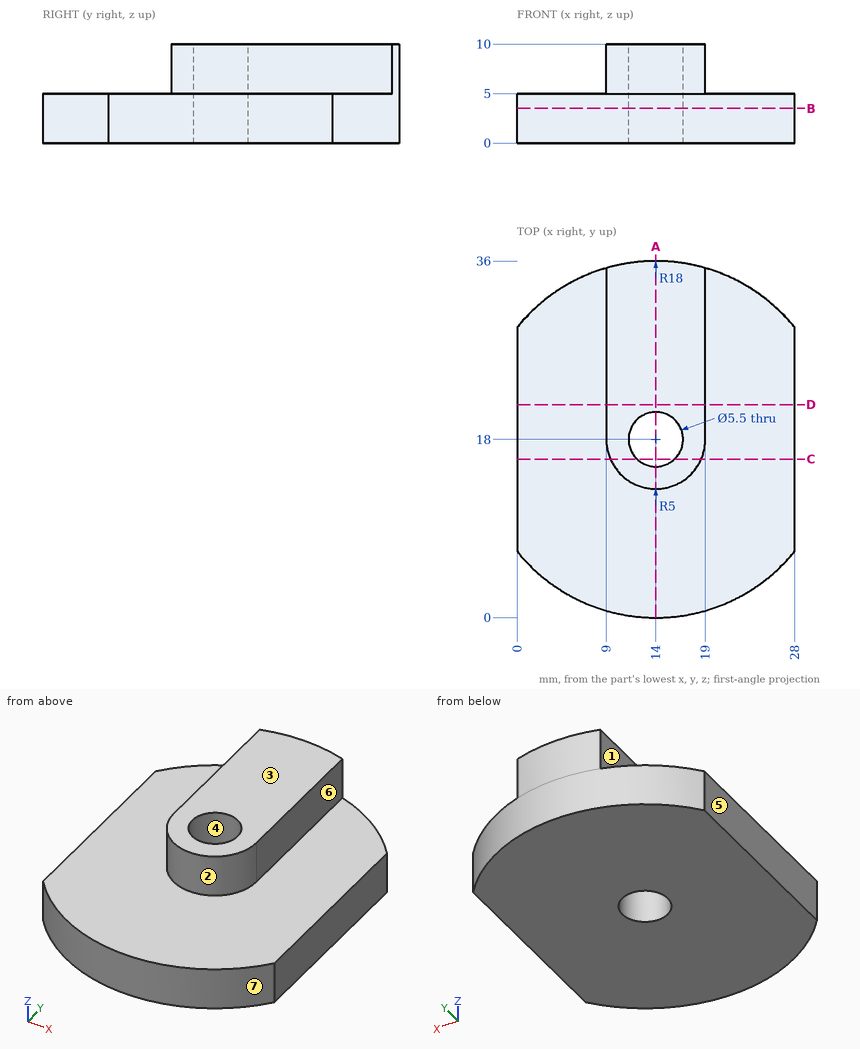
Check sheet for the drawn part. Datum: minimum x, y, z corner. Units: mm. A direction names the side the tool comes from. Round coordinates to 2 decimals unless told otherwise and drop trailing zeros. Order: outer loops, then holes, each group sorted by start corner. A loop starts at its lowest first (then second) coordinate and runs counter-clockwise, first axis right, second up. Notation, with made-up numbers: M 48,46 L 70,46 A14 cw 70,64 Z; hole C -34,23.5 d2. An arc over 180 degrees is marked long. Answer in a Markdown table with one row per item.
(1) Section check D-D on y = 21.5. Record the boundary of the cut face in (x, z), plus the area to 3 significant figures.
Findings:
| item | result |
|---|---|
| outline | M 0,0 L 28,0 L 28,5 L 19,5 L 19,10 L 9,10 L 9,5 L 0,5 Z |
| area | 190 mm^2 |
(2) Material ranges on line 1 along X through (y, z) = (18, 3); line 2 along Y through (x, z) = (14, 2.5); line 3 along Y through (x, z) = (14, 6.25), recorded low to high. Write a range as from..to.
Findings:
| item | result |
|---|---|
| line 1 | x = 0..11.25, 16.75..28 |
| line 2 | y = 0..15.25, 20.75..36 |
| line 3 | y = 13..15.25, 20.75..36 |
(3) Set-up check for the marked faces 1, 2 and 3: record each of +Z, -Z, +X, -X, +Y, -Y from which the full face is reachable in a straight line by a thin tool's end or side.
Findings:
| item | result |
|---|---|
| face 1 | +Z, -X, +Y, -Y |
| face 2 | +Z, -Y |
| face 3 | +Z, +X, -X, +Y, -Y |
(4) Section check C-C on y = 16. Record the boundary of the cut face in (x, z).
Findings:
| item | result |
|---|---|
| outline | M 0,0 L 12.11,0 L 12.11,10 L 9.42,10 L 9.42,5 L 0,5 Z; M 15.89,0 L 28,0 L 28,5 L 18.58,5 L 18.58,10 L 15.89,10 Z |
(5) Section check B-B on z = 3.5. Record the boundary of the cut face in (x, y).
Findings:
| item | result |
|---|---|
| outline | M 0,6.69 A18 ccw 28,6.69 L 28,29.31 A18 ccw 0,29.31 Z; hole C 14,18 d5.5 |
(6) Draft check along X on the marked faces 4, 5, 6 and 7. Enter one of: +X half, -X half, draft (parallel to the pull), parting line (faces both ways), or undercut.
Findings:
| item | result |
|---|---|
| face 4 | undercut |
| face 5 | -X half |
| face 6 | +X half |
| face 7 | parting line |
(7) Gauge pin test, flat ends, axial feed: pin 1 (1 mm diameter, centred on x = 24.5, z = 3.5, fed in from +Y); pin 2 (1.5 mm diameter, centred on y = 27.5, z = 7.5, fed in from +X); pin 3 (1.5 mm diameter, centred on y = 26.5, z = 7.5, fed in from -X); pin 4 (3.5 mm diameter, centred on x = 14, y = 18, fed in from -Z). Record the tip position at first contact, or that the pin passes through.
Findings:
| item | result |
|---|---|
| pin 1 | stops at y = 32.97 |
| pin 2 | stops at x = 19 |
| pin 3 | stops at x = 9 |
| pin 4 | passes through |
(8) Section check A-A on x = 14. Record the boundary of the cut face in (y, z), plus the area to 3 significant figures.
Findings:
| item | result |
|---|---|
| outline | M 0,0 L 15.25,0 L 15.25,10 L 13,10 L 13,5 L 0,5 Z; M 20.75,0 L 36,0 L 36,10 L 20.75,10 Z |
| area | 240 mm^2 |
